from build123d import *

# Parameters (mm, degrees)
F0_R      = 7.9375
F1_DEPTH  = 1.5875
F2_R      = 7.4676
F3_DEPTH  = 1.016
F4_R      = 7.9375
F5_DEPTH  = 50.8
F6_R      = 7.4676
F7_DEPTH  = 1.016
F8_R      = 7.9375
F9_DEPTH  = 4.7625
F10_R     = 7.4676
F11_DEPTH = 1.016
F12_R     = 7.9375
F13_DEPTH = 65.0875
F14_R     = 7.4676
F15_DEPTH = 1.016
F16_R     = 7.9375
F17_DEPTH = 186.309
F18_R     = 7.4676
F19_DEPTH = 1.016
F20_R     = 7.9375
F21_DEPTH = 9.525
F22_R     = 7.4676
F23_DEPTH = 1.016
F24_R     = 7.9375
F25_DEPTH = 1.5875
F26_SIZE  = 0.79375


with BuildPart() as f1:
    # F0 (on Front) → F1 (new body)
    with BuildSketch(Plane.XZ):
        Circle(F0_R)
    extrude(amount=F1_DEPTH)

    # F2 (on face) → F3 (join)
    with BuildSketch(Plane.XZ.offset(1.5875)):
        Circle(F2_R)
    extrude(amount=F3_DEPTH)

    # F4 (on face) → F5 (join)
    with BuildSketch(Plane.XZ.offset(2.6035)):
        Circle(F4_R)
    extrude(amount=F5_DEPTH)

    # F6 (on face) → F7 (join)
    with BuildSketch(Plane.XZ.offset(53.4035)):
        Circle(F6_R)
    extrude(amount=F7_DEPTH)

    # F8 (on face) → F9 (join)
    with BuildSketch(Plane.XZ.offset(54.4195)):
        Circle(F8_R)
    extrude(amount=F9_DEPTH)

    # F10 (on face) → F11 (join)
    with BuildSketch(Plane.XZ.offset(59.182)):
        Circle(F10_R)
    extrude(amount=F11_DEPTH)

    # F12 (on face) → F13 (join)
    with BuildSketch(Plane.XZ.offset(60.198)):
        Circle(F12_R)
    extrude(amount=F13_DEPTH)

    # F14 (on face) → F15 (join)
    with BuildSketch(Plane.XZ.offset(125.2855)):
        Circle(F14_R)
    extrude(amount=F15_DEPTH)

    # F16 (on face) → F17 (join)
    with BuildSketch(Plane.XZ.offset(126.3015)):
        Circle(F16_R)
    extrude(amount=F17_DEPTH)

    # F18 (on face) → F19 (join)
    with BuildSketch(Plane.XZ.offset(312.6105)):
        Circle(F18_R)
    extrude(amount=F19_DEPTH)

    # F20 (on face) → F21 (join)
    with BuildSketch(Plane.XZ.offset(313.6265)):
        Circle(F20_R)
    extrude(amount=F21_DEPTH)

    # F22 (on face) → F23 (join)
    with BuildSketch(Plane.XZ.offset(323.1515)):
        Circle(F22_R)
    extrude(amount=F23_DEPTH)

    # F24 (on face) → F25 (join)
    with BuildSketch(Plane.XZ.offset(324.1675)):
        Circle(F24_R)
    extrude(amount=F25_DEPTH)

    # F26
    f26_edges = [f1.edges().sort_by_distance(p)[0] for p in [
        (-7.9375, -325.755, 0),
        (-7.9375, 0, 0),
    ]]
    chamfer(f26_edges, length=F26_SIZE)


solid = f1.part
Geometry: final body of the model. Coordinates: model frame, mm. A direction names the side the tool comes from. Give positions to 0.01 mm unless a question says otherwise; leave off trailing zeros. Order: outer loops, then holes, each group sorted by start corner. A loop starts at its lowest first (then second) coordinate and runs counter-clockwise, first axis right, second up. Notation, with made-up numbers: (58.25, -1) -> (116.25, -1) arc R14 cw to (116.25, 16) -> close; hole circle Ø5 at (-33.5, 52). An arc over 180 degrees is marked (long way). Answer as a JSON object with one key per item and string values.
Q1. Draft query along Y for faces 3 (the flat face through (0, -325.755, 0)), 4 (the cylindrical face through (-1.62, -323.65, -7.29)), 5 (the cylindrical face through (-1.72, -27.65, -7.75)). Return one class per face: released by +Y, released by -Y, zero draft, split by the parting line, or undercut.
Entries:
{"face 3": "released by -Y", "face 4": "undercut", "face 5": "zero draft"}
Q2. Material intervals for probe 1 along Z at (x, y) = (-0.75, -45.5); probe 2 along Z at (x, y) = (3.5, -115); probe 3 along X at (y, z) = (-288, -0.25), sorted ascending.
Entries:
{"probe 1": "z = -7.9 to 7.9", "probe 2": "z = -7.12 to 7.12", "probe 3": "x = -7.93 to 7.93"}
Q3. Section A-A (y = -286.5). Output: boundary loops of the cut face in (x, z) (1 decimal), plus the area to 3 significant figures.
Entries:
{"outline": "circle Ø15.9 at (0, 0)", "area": "198 mm^2"}
Q4. Access query for faces 1 (the cylindrical face through (-1.72, -218.15, -7.75)), 2 (the cylindrical face through (-1.62, -2.09, -7.29)). Directions: +Z, -Z, +X, -X, +Y, -Y. A direction counts if a zero-diameter tool reaches every point of the face in a straight line with its end or side. Return the directions, or none.
Entries:
{"face 1": "+Y, -Y", "face 2": "none"}
Q5. First-contact query: pin 1 (5 mm diameter, centred on y = -71, z = -3.5, fed in from +X); pin 2 (1 mm diameter, centred on y = -172, z = -1, fed in from -X); pin 3 (1.5 mm diameter, centred on x = -3.5, y = -151, fed in from -Z). Flat tips, straight axial feed; report the tip coordinate or a pass-through.
Entries:
{"pin 1": "stops at x = 7.87", "pin 2": "stops at x = -7.92", "pin 3": "stops at z = -7.45"}
